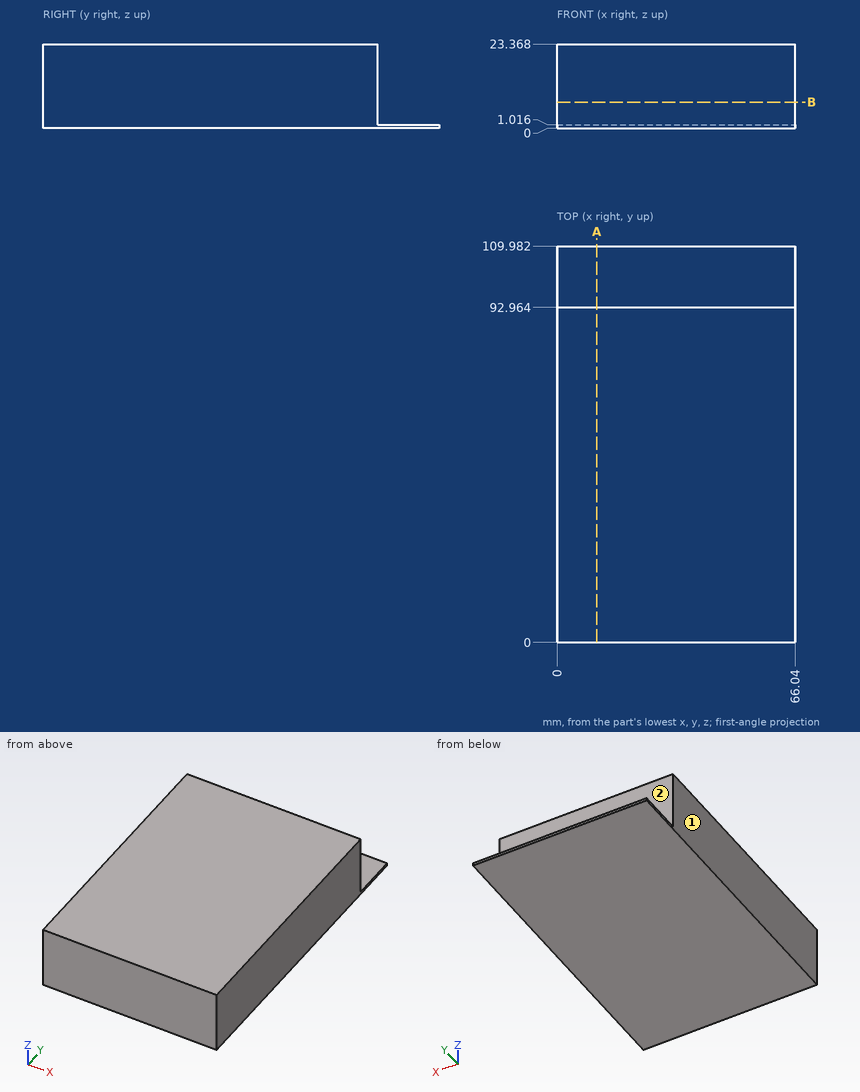
Print and shaded views of the part. All mm, measured from the part's lowest x, y and z. A direction names the side the tool comes from. Give positions to 0.01 mm unless a question says otherwise; leave off trailing zeros. Order: outer loops, then holes, each group sorted by start corner. A loop starts at its lowest first (then second) coordinate and runs counter-clockwise, first axis right, second up. Notation, with made-up numbers: (50.25, 3.5) - (84.25, 3.5) arc R12 ccw to (84.25, 24.5) - close; hole circle Ø1 at (65.5, 68). An arc over 180 degrees is marked (long way). One line per item, written item: value.
Item 1: Slice it at B-B (z = 7.25). List the corners of the cut face in (x, y).
Response values:
outline: (0, 0) - (66.04, 0) - (66.04, 92.96) - (0, 92.96) - close
Item 2: Wall check: line 1 (Y direction, x = 45, z = 4). Give the ranges that are in metal, low to high.
Response values:
line 1: 0 to 92.96
Item 3: Slice it at A-A (x = 11). List the corners of the cut face in (y, z), then the cut area to 3 significant figures.
Response values:
outline: (0, 0) - (109.98, 0) - (109.98, 1.02) - (92.96, 1.02) - (92.96, 23.37) - (0, 23.37) - close
area: 2,190 mm2
Item 4: Tool access for the marked faces 1 and 2: list every direction of +Z, -Z, +X, -X, +Y, -Y with a clear straight run to the whole face (end or side of a thin tool).
Response values:
face 1: +Z, -Z, -X, +Y, -Y
face 2: +Z, +X, -X, +Y
Item 5: Pin check, flat tips, straight feed: pin 1 Ø12 at (x, y) = (27.5, 15.5) entering from -Z; pin 2 Ø8.5 at (x, y) = (41.5, 105.5) entering from +Z; pin 3 Ø1 at (x, z) = (57.5, 18.5) entering from +Y. Stop position of each tip, or through.
Response values:
pin 1: z = 0
pin 2: z = 1.02
pin 3: y = 92.96
